The figure shows three views and two pictorial views of one solid part (mm, origin at its lowest corner). Answer the questions. Coordinates: 2 decimals unless noted, no trailing zeros. Loops run counter-clockwise (first coordinate to the right, second up) from the corner with the lowest first, then second, coordinate; pieces in that order, holes last. Notation, with made-up numbers: M 20,16.5 L 51,16.5 A15 cw 51,38.5 Z; hole C 80,30 d6. An arc over 180 degrees is marked long. Return JSON: item names as keys, results as strings. Group by question number.
1. Section A-A (x = 3.18) is taken. Write down the section's boundary in (y, z), then the cut area to 3 significant figures.
2. Section C-C (z = 1.85) is taken. Write down the section's boundary in (x, y), then the cut area to 3 significant figures.
3. Straight lines are drawn through the part: L1, parallel to Z at x = 3.18, y = 9; L2, parallel to X at y = 9, z = 2.15; L3, parallel to Z at x = 3.5, y = 7.25. For each, find the intervals that lie inside material, in ascending order. Write a range as from..to.
4. The mould has two halves that part along Z. Classify the marked faces 1, 2 and 3: pulls with the +Z half, pulls with the -Z half, needs draft (parallel to the pull), parting line crosses it, or undercut.
5. Section D-D (x = 1) is taken. Write down the section's boundary in (y, z), then the cut area to 3 significant figures.
6. Given P1, Ø2, axis at y = 2, z = 1.5, coming from the +X side, flat-ended and moving along its own axis, determine where the tip first touches the part or whether it passes through.
7. Section B-B (y = 5.75) is taken. Write down the section's boundary in (x, z).
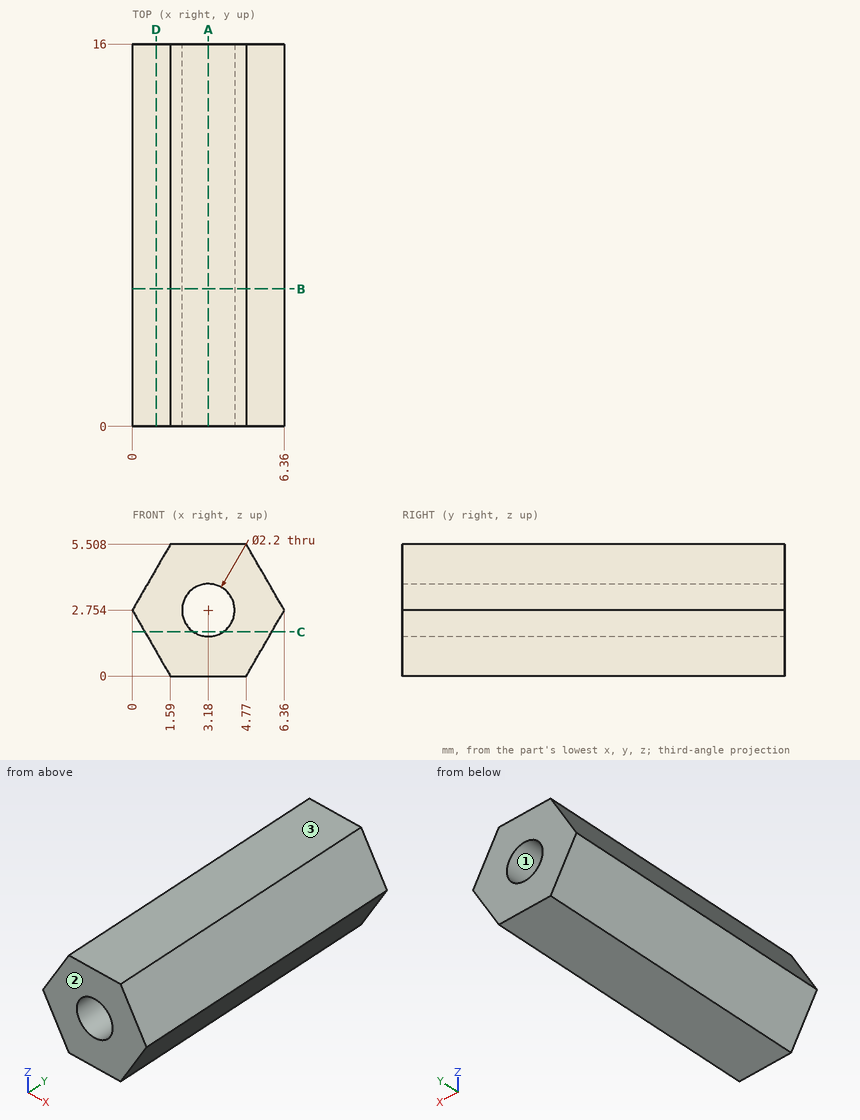
Worked out:
{
 "1": {"outline": "M 0,0 L 16,0 L 16,1.65 L 0,1.65 Z; M 0,3.85 L 16,3.85 L 16,5.51 L 0,5.51 Z", "area": "52.9 mm^2"},
 "2": {"outline": "M 0.52,0 L 2.55,0 L 2.55,16 L 0.52,16 Z; M 3.81,0 L 5.84,0 L 5.84,16 L 3.81,16 Z", "area": "65.0 mm^2"},
 "3": {"L1": "0..1.65, 3.85..5.51", "L2": "0.35..2.26, 4.1..6.01", "L3": "0..1.7, 3.81..5.51"},
 "4": {"face 1": "undercut", "face 2": "needs draft", "face 3": "pulls with the +Z half"},
 "5": {"outline": "M 0,1.02 L 16,1.02 L 16,4.49 L 0,4.49 Z", "area": "55.4 mm^2"},
 "6": {"P1": "x = 6.21"},
 "7": {"outline": "M 0,2.75 L 1.59,0 L 4.77,0 L 6.36,2.75 L 4.77,5.51 L 1.59,5.51 Z; hole C 3.18,2.75 d2.2"}
}
